from build123d import *

# Parameters (mm, degrees)
SKETCH1_W           = 200
SKETCH1_H           = 120
BOSS_EXTRUDE1_DEPTH = 3
SKETCH2_W           = 200
SKETCH2_H           = 120
BOSS_EXTRUDE2_DEPTH = 37


with BuildPart() as part:
    # Sketch1 → Boss-Extrude1 (new body)
    with BuildSketch(Plane(origin=(0, 0, 0), x_dir=(1, 0, 0), z_dir=(0, 1, 0))):
        with Locations((100, 60)):
            Rectangle(SKETCH1_W, SKETCH1_H)
    extrude(amount=BOSS_EXTRUDE1_DEPTH)

    # Sketch2 → Boss-Extrude2 (add)
    with BuildSketch(Plane(origin=(0, 3, 0), x_dir=(1, 0, 0), z_dir=(0, 1, 0))):
        with Locations((100, 60)):
            Rectangle(SKETCH2_W, SKETCH2_H)
        with BuildLine():
            Line((3, 98.3), (3, 21.7))
            ThreePointArc((3, 21.7), (9.01040764, 19.21040764), (11.5, 13.2))
            Line((11.5, 13.2), (11.5, 3))
            Line((11.5, 3), (188.5, 3))
            Line((188.5, 3), (188.5, 13.2))
            ThreePointArc((188.5, 13.2), (190.98959236, 19.21040764), (197, 21.7))
            Line((197, 21.7), (197, 98.3))
            ThreePointArc((197, 98.3), (190.98959236, 100.78959236), (188.5, 106.8))
            Line((188.5, 106.8), (188.5, 117))
            Line((188.5, 117), (11.5, 117))
            Line((11.5, 117), (11.5, 106.8))
            ThreePointArc((11.5, 106.8), (9.01040764, 100.78959236), (3, 98.3))
        make_face(mode=Mode.SUBTRACT)
    extrude(amount=BOSS_EXTRUDE2_DEPTH)


solid = part.part
Here's how the part is built. I have some questions about the finished solid (model axes, mm). A direction names the side the tool comes from. Coordinates: 2 decimals unless noted, no trailing zeros. Loops run counter-clockwise (first coordinate to the right, second up) from the corner with the lowest first, then second, coordinate; pieces in that order, holes last.
1. For faces 1 (the flat face through (99, 0, -61)), 2 (the flat face through (197, 21, -59)), which set-ups out of +Z, -Z, +X, -X, +Y, -Y let a thin tool reach every point of the face, with its end or its side?
2. If we mould it in two halves opening along X, with no side actions, what happens to faces 3 (the flat face through (0, 20, -59)), 4 (the flat face through (99, 20, 0)), 5 (the cylindrical face through (8.94, 21.24, -19.28))? For each: pulls with the +X half, pulls with the -X half, needs draft (parallel to the pull), parting line crosses it, or undercut.
3. Imagine slicing it at B-B, the plane z = -73.5. Please give me the cut outline in (x, y).
4. Imagine slicing it at C-C, the plane x = 92.5. Please give me the cut outline in (y, z).
5. For P1, Ø4, axis at x = 29.5, z = -89.5, coming from the +Y side; P2, Ø3, axis at y = 19, z = -110.5, coming from the -X side, each with a flat end and sliding along its axis, tell me the tip position at first contact or that it passes through.
6. I need wall thicknesses on L1, parallel to Z at x = 117, y = 6; L2, parallel to X at y = 27.5, z = -73; L3, parallel to Y at x = 99, z = -41.5. Which ranges of each line are inside material? Lowest first, please.
7. Imagine slicing it at A-A, the plane y = 23.5. Please give me the cut outline in (x, z).
Taken from the geometry:
1. face 1: +Z, -Z, +X, -X, -Y
1. face 2: +Y
2. face 3: pulls with the -X half
2. face 4: needs draft
2. face 5: undercut
3. outline: (0, 0) - (200, 0) - (200, 40) - (197, 40) - (197, 3) - (3, 3) - (3, 40) - (0, 40) - close
4. outline: (0, -120) - (40, -120) - (40, -117) - (3, -117) - (3, -3) - (40, -3) - (40, 0) - (0, 0) - close
5. P1: stops at y = 3
5. P2: stops at x = 0
6. L1: z = -120 to -117, -3 to 0
6. L2: x = 0 to 3, 197 to 200
6. L3: y = 0 to 3
7. outline: (0, -120) - (200, -120) - (200, 0) - (0, 0) - close; hole (3, -98.3) arc R8.5 cw to (11.5, -106.8) - (11.5, -117) - (188.5, -117) - (188.5, -106.8) arc R8.5 cw to (197, -98.3) - (197, -21.7) arc R8.5 cw to (188.5, -13.2) - (188.5, -3) - (11.5, -3) - (11.5, -13.2) arc R8.5 cw to (3, -21.7) - close
